Input: dimensioned drawing with shaded views. Units: mm. Origin: part minimum x, y, z. A direction names the side the tool comes from. Coordinates: 2 decimals unless noted, no trailing zeros. Loops run counter-clockwise (first coordinate to the right, second up) from the corner with the lowest first, then second, coordinate; pieces in that order, holes last. Notation, with made-up numbers: (1.5, 38) -> (15.5, 38) arc R29 ccw to (15.5, 67) -> close; hole circle Ø11 at (65, 63). An arc over 180 degrees is marked (long way). Answer as CSV lines item,"result".
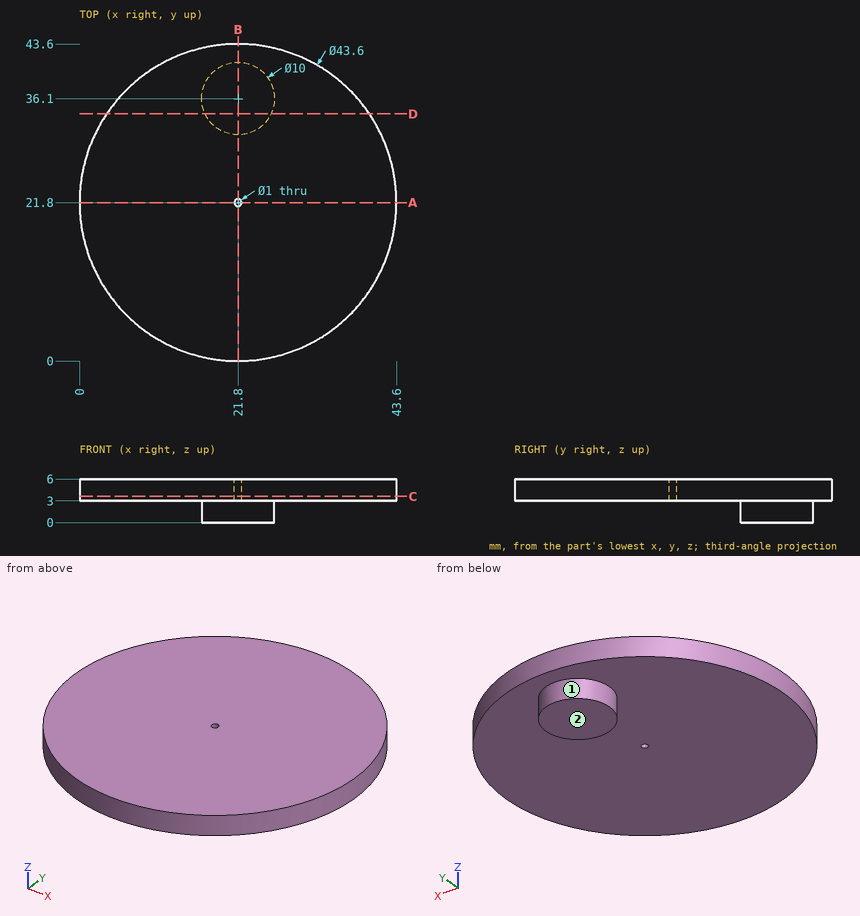
(1) Cut plane D-D (y = 34). Return the cut outline in (x, z).
Computed values:
outline,"(3.73, 3) -> (17.26, 3) -> (17.26, 0) -> (26.34, 0) -> (26.34, 3) -> (39.87, 3) -> (39.87, 6) -> (3.73, 6) -> close"
(2) Pin query (flat end, axial travel): pin 1 Ø8 at (x, y) = (38, 19) entering from -Z; pin 2 Ø1 at (y, z) = (34, 1.5) entering from +X; pin 3 Ø1.5 at (y, z) = (9.5, 5) entering from -X. Return the tip coordinate at first contact, or that it passes through.
Computed values:
pin 1,"z = 3"
pin 2,"x = 26.54"
pin 3,"x = 3.31"
(3) Cut plane C-C (z = 3.6). Return the cut outline in (x, y).
Computed values:
outline,"circle Ø43.6 at (21.8, 21.8); hole circle Ø1 at (21.8, 21.8)"
(4) Material intervals for L1, parallel to Y at x = 21.8, z = 3.95; L2, parallel to Z at x = 26.5, y = 2; L3, parallel to Y at x = 41, z = 5.05, sorted ascending. Write a range as [from, to].
Computed values:
L1,"[0, 21.3], [22.3, 43.6]"
L2,"[3, 6]"
L3,"[11.48, 32.12]"
(5) Access query for the marked faces 1 and 2. Directions: +Z, -Z, +X, -X, +Y, -Y. A direction counts if a zero-diameter tool reaches every point of the face in a straight line with its end or side. Return the directions, or none.
Computed values:
face 1,"-Z"
face 2,"-Z, +X, -X, +Y, -Y"
(6) Cut plane B-B (x = 21.8). Return the cut outline in (y, z), then the cut area to 3 significant figures.
Computed values:
outline,"(0, 3) -> (21.3, 3) -> (21.3, 6) -> (0, 6) -> close; (22.3, 3) -> (31.1, 3) -> (31.1, 0) -> (41.1, 0) -> (41.1, 3) -> (43.6, 3) -> (43.6, 6) -> (22.3, 6) -> close"
area,"158 mm^2"
(7) Cut plane A-A (y = 21.8). Return the cut outline in (x, z), then the cut area to 3 significant figures.
Computed values:
outline,"(0, 3) -> (21.3, 3) -> (21.3, 6) -> (0, 6) -> close; (22.3, 3) -> (43.6, 3) -> (43.6, 6) -> (22.3, 6) -> close"
area,"128 mm^2"
